Could you check a few things on this model? Use its own coordinates, in mm. Give positions to 0.01 mm unless a question says otherwise; leave off trailing zeros. Write each loop counter-clockwise with the first axis right and the second up, starting at its lowest first coordinate (ties: lowest second). Pieces come first, ordered by that corner, then holes. Notation, with made-up numbers: (43.25, 19) - (79.25, 19) arc R8 ccw to (79.25, 23) - close; hole circle Ø2 at (45.5, 26). An arc over 180 degrees is marked (long way). Write item = value, one per line.
from build123d import *

# Parameters (mm, degrees)
F1_DEPTH = 10
F2_R     = 5
F3_R     = 5
F4_SIZE  = 5


with BuildPart() as f1:
    # F0 (on Top) → F1 (new body)
    with BuildSketch(Plane.XY):
        Polygon((-15.45085, 21.26627), (-25, -8.122992), (25, -8.122992), (15.45085, 21.26627), align=None)
    extrude(amount=F1_DEPTH)

    # F2
    f2_edges = [f1.edges().sort_by_distance(p)[0] for p in [
        (15.45085, 21.26627, 5),
    ]]
    fillet(f2_edges, radius=F2_R)

    # F3
    f3_edges = [f1.edges().sort_by_distance(p)[0] for p in [
        (-15.45085, 21.26627, 5),
    ]]
    fillet(f3_edges, radius=F3_R)

    # F4
    f4_edges = [f1.edges().sort_by_distance(p)[0] for p in [
        (0, 21.26627, 10),
        (-14.757063, 20.311355, 10),
        (14.757063, 20.311355, 10),
        (-20.78671, 4.844181, 10),
        (20.78671, 4.844181, 10),
        (0, -8.122992, 10),
    ]]
    chamfer(f4_edges, length=F4_SIZE)


solid = f1.part
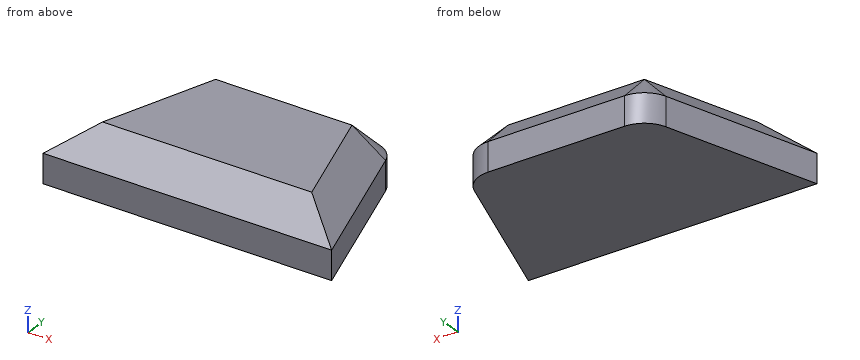
1. If we section it at C-C, the plane x = 20.5: Please give me the cut outline in (y, z), and give its area (3 significant figures).
Filled sheet:
outline = (-8.12, 0) - (5.73, 0) - (5.73, 5) - (-4.85, 8.27) - (-8.12, 5) - close
area = 91.9 mm2
2. I need wall thicknesses on line 1 (Z direction, x = 12.5, y = 14.5); line 2 (X direction, y = 13.5, z = 3.5); line 3 (Y direction, x = -9.5, z = 5.5). Which ranges of each line are inside material? Lowest first, please.
Filled sheet:
line_1 = 0 to 9.9
line_2 = -17.97 to 17.97
line_3 = -7.62 to 20.77
3. For pin 1 (1.5 mm diameter, centred on y = 7.5, z = 5, fed in from -X); pin 2 (2 mm diameter, centred on x = -10, z = 8.5, fed in from -Y); pin 3 (1.5 mm diameter, centred on y = 7, z = 1, fed in from -X), each with a flat end and sliding along its axis, tell me the tip position at first contact or that it passes through.
Filled sheet:
pin_1 = -20.17
pin_2 = -5.62
pin_3 = -20.33
4. If we section it at B-B, the plane x = -8: Please give me the cut outline in (y, z).
Filled sheet:
outline = (-8.12, 0) - (21.27, 0) - (21.27, 5) - (16.27, 10) - (-3.12, 10) - (-8.12, 5) - close
5. If we section it at A-A, the plane z = 4: Please give me the cut outline in (x, y).
Filled sheet:
outline = (-25, -8.12) - (25, -8.12) - (16.57, 17.81) arc R5 ccw to (11.82, 21.27) - (-11.82, 21.27) arc R5 ccw to (-16.57, 17.81) - close
